Geometry check sheet. Reference: the model listing, model coordinates, mm. Face numbers are marked on the shaded views. A direction names the side the tool comes from. Coordinates: 2 decimals unless noted, no trailing zeros. Write each loop counter-clockwise with the first axis right and the second up, starting at its lowest first coordinate (ties: lowest second). Pieces come first, ordered by that corner, then holes. Notation, with made-up numbers: (-21.5, -17.75) -> (26.5, -17.75) arc R13 cw to (26.5, 0.25) -> close; hole circle Ø8 at (58, 38.25). An arc over 180 degrees is marked (long way). Use a Markdown table: item, result.
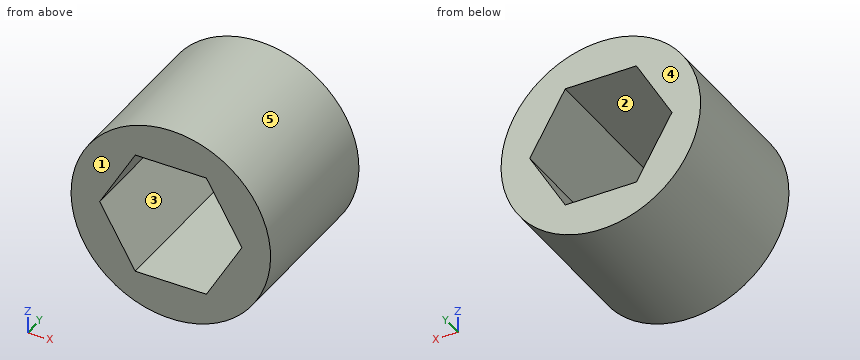
```python
from build123d import *

# Parameters (mm, degrees)
SKETCH1_R           = 5.75
SKETCH1_R_2         = 4.1
BOSS_EXTRUDE1_DEPTH = 9


with BuildPart() as part:
    # Sketch1 → Boss-Extrude1 (new body)
    with BuildSketch(Plane(origin=(0, 0, 0), x_dir=(1, 0, 0), z_dir=(0, 1, 0))):
        with Locations(Location((0, 0, 0), (0, 0, 270))):
            Circle(SKETCH1_R)
        Circle(SKETCH1_R_2, mode=Mode.SUBTRACT)
        with BuildLine():
            ThreePointArc((-2.05, -3.550704156), (0, -4.1), (2.05, -3.550704156))
            Line((2.05, -3.550704156), (-2.05, -3.550704156))
        make_face()
        with BuildLine():
            Line((4.1, 0), (2.05, -3.550704156))
            ThreePointArc((2.05, -3.550704156), (3.550704156, -2.05), (4.1, 0))
        make_face()
        with BuildLine():
            Line((2.05, 3.550704156), (4.1, 0))
            ThreePointArc((4.1, 0), (3.550704156, 2.05), (2.05, 3.550704156))
        make_face()
        with BuildLine():
            Line((-2.05, 3.550704156), (2.05, 3.550704156))
            ThreePointArc((2.05, 3.550704156), (0, 4.1), (-2.05, 3.550704156))
        make_face()
        with BuildLine():
            ThreePointArc((-2.05, 3.550704156), (-3.550704156, 2.05), (-4.1, 0))
            Line((-4.1, 0), (-2.05, 3.550704156))
        make_face()
        with BuildLine():
            ThreePointArc((-4.1, 0), (-3.550704156, -2.05), (-2.05, -3.550704156))
            Line((-2.05, -3.550704156), (-4.1, 0))
        make_face()
    extrude(amount=BOSS_EXTRUDE1_DEPTH)


solid = part.part
```
Item 1: Section check D-D on x = 4.5. Record the boundary of the cut face in (y, z).
Answer block:
| item | result |
|---|---|
| outline | (0, -3.58) -> (9, -3.58) -> (9, 3.58) -> (0, 3.58) -> close |
Item 2: Depth check by flat-ended pin: P1, Ø1, axis at x = 1, z = -1.5, coming from the +Y side; P2, Ø1, axis at y = 4.5, z = 4.5, coming from the -X side; P3, Ø1, axis at y = 2.5, z = -4, coming from the -X side; P4, Ø1.5, axis at x = 1.5, y = 4, coming from the -Z side. Enter the tip coordinate at first touch or a pass-through.
Answer block:
| item | result |
|---|---|
| P1 | passes through |
| P2 | stops at x = -4.13 |
| P3 | stops at x = -4.56 |
| P4 | stops at z = -5.7 |
Item 3: Tool access check on the marked faces 1 and 2. Record the directions out of +Z, -Z, +X, -X, +Y, -Y that give a thin tool (end or side, any length) a straight path to the whole face; none if there is none.
Answer block:
| item | result |
|---|---|
| face 1 | +Z, -Z, +X, -X, -Y |
| face 2 | +Y, -Y |
Item 4: Section check C-C on z = 0.5. Record the boundary of the cut face in (x, y), then the cut area to 3 significant figures.
Answer block:
| item | result |
|---|---|
| outline | (-5.73, 0) -> (-3.81, 0) -> (-3.81, 9) -> (-5.73, 9) -> close; (3.81, 0) -> (5.73, 0) -> (5.73, 9) -> (3.81, 9) -> close |
| area | 34.5 mm^2 |
Item 5: Mould release check, pull along Z, two halves, no side actions. Record for the marked faces 3, 4 and 5: +Z half, -Z half, draft (parallel to the pull), parting line (faces both ways), or undercut.
Answer block:
| item | result |
|---|---|
| face 3 | undercut |
| face 4 | draft |
| face 5 | parting line |
Item 6: Section check A-A on x = 0. Record the boundary of the cut face in (y, z), then the cut area to 3 significant figures.
Answer block:
| item | result |
|---|---|
| outline | (0, -5.75) -> (9, -5.75) -> (9, -3.55) -> (0, -3.55) -> close; (0, 3.55) -> (9, 3.55) -> (9, 5.75) -> (0, 5.75) -> close |
| area | 39.6 mm^2 |
Item 7: Section check B-B on y = 2.75. Record the boundary of the cut face in (x, z), then the cut area to 3 significant figures.
Answer block:
| item | result |
|---|---|
| outline | circle Ø11.5 at (0, 0); hole (-4.1, 0) -> (-2.05, -3.55) -> (2.05, -3.55) -> (4.1, 0) -> (2.05, 3.55) -> (-2.05, 3.55) -> close |
| area | 60.2 mm^2 |
Item 8: Thickness scan on L1, parallel to Z at x = -2, y = 4.5; L2, parallel to X at y = 3.25, z = -2; L3, parallel to Z at x = 3, y = 7.25. Record the ranges inside material, lowest first. Write a range as [from, to].
Answer block:
| item | result |
|---|---|
| L1 | z = [-5.39, -3.55], [3.55, 5.39] |
| L2 | x = [-5.39, -2.95], [2.95, 5.39] |
| L3 | z = [-4.91, -1.91], [1.91, 4.91] |
